```python
from build123d import *

# Parameters (mm, degrees)
F0_W      = 1200
F0_H      = 800
F1_DEPTH  = 60
F4_DEPTH  = 25
F5_W      = 1136.9413696229
F5_H      = 692.619483918
F6_DEPTH  = 30
F7_W      = 1159.0888965875
F7_H      = 738.1461262703
F8_DEPTH  = 15
F9_W      = 180.6832998991
F9_H      = 355.1081307232
F9_W_2    = 16.8206766248
F9_W_3    = 982.4556671083
F9_H_2    = 21.863527596
F9_H_3    = 568.6533860862
F10_DEPTH = 15


# Not quite as in the source:
# - the program builds the solid bodies; features that only make, move or delete a surface that nothing else refers to are left out


with BuildPart() as f1:
    # F0 (on Top) → F1 (new body)
    with BuildSketch(Plane.XY):
        with Locations((600, 400)):
            Rectangle(F0_W, F0_H)
    extrude(amount=F1_DEPTH)

    # F4 (add): a face of the model
    f4_faces = [f1.faces().sort_by_distance(p)[0] for p in [
        (600, 400, 0),
    ]]
    extrude(f4_faces, amount=F4_DEPTH)

    # F5 (on face) → F6 (cut)
    with BuildSketch(Plane(origin=(0, 0, -25), x_dir=(1, 0, 0), z_dir=(0, 0, -1))):
        with Locations((594.3454820663, -399.9507818371)):
            Rectangle(F5_W, F5_H)
    extrude(amount=-F6_DEPTH, mode=Mode.SUBTRACT)

    # F7 (on face) → F8 (cut)
    with BuildSketch(Plane.XY.offset(60)):
        with Locations((602.350092493, 395.9690630436)):
            Rectangle(F7_W, F7_H)
    extrude(amount=-F8_DEPTH, mode=Mode.SUBTRACT)

    # F9 (on face) → F10 (cut)
    with BuildSketch(Plane(origin=(0, 0, -25), x_dir=(1, 0, 0), z_dir=(0, 0, -1))):
        with Locations((-90.3416499496, -193.3716591448)):
            Rectangle(F9_W, F9_H)
        with Locations((8.4103383124, -193.3716591448)):
            Rectangle(F9_W_2, F9_H)
        with Locations((517.1026308089, -42.7092760801)):
            Rectangle(F9_W_3, F9_H_2)
        Polygon((1162.8161668777, -53.6410398781), (1008.3304643631, -53.6410398781), (1008.3304643631, -622.2944259644), (25.8747972548, -622.2944259644), (25.8747972548, -746.2605237961), (1162.8161668777, -746.2605237961), align=None)
        with Locations((517.1026308089, -337.9677329212)):
            Rectangle(F9_W_3, F9_H_3)
        Polygon((25.8747972548, -15.8175937831), (25.8747972548, -31.7775122821), (1008.3304643631, -31.7775122821), (1008.3304643631, -53.6410398781), (1162.8161668777, -53.6410398781), (1162.8161668777, -746.2605237961), (25.8747972548, -746.2605237961), (25.8747972548, -781.8935513496), (1179.8995733261, -781.8935513496), (1179.8995733261, -15.8175937831), align=None)
    extrude(amount=-F10_DEPTH, mode=Mode.SUBTRACT)


solid = f1.part
```
Check sheet for the modelled part. Datum: model origin and axes. Units: mm. A direction names the side the tool comes from. Give positions to 0.01 mm unless a question says otherwise; leave off trailing zeros. Order: outer loops, then holes, each group sorted by start corner. A loop starts at its lowest first (then second) coordinate and runs counter-clockwise, first axis right, second up. Notation, with made-up numbers: M -6,21 L 14,21 A25 ccw 14,47 Z; hole C 27.25,62 d1. An arc over 180 degrees is marked long. Answer in a Markdown table with one row per item. Add a question column.
Q1. Gauge pin test, flat ends, axial feed: pin 1 Ø7.5 at (y, z) = (231.5, -14) entering from -X; pin 2 Ø8 at (x, y) = (374.5, 261.5) entering from +Z. Record the tip position at first contact, or that the pin passes through.
Q2. Release check for a two-part mould opening along X. For faces 4 (the flat face through (592, 800, 18)), 5 (the flat face through (586, 395, 5)), 6 (the flat face through (25.875, 404, -10)), 7 (the flat face through (1200, 394, 18)) record: released by +X, released by -X, zero draft, split by the parting line, or undercut.
Q3. Thickness scan on L1, parallel to X at y = 310.5, z = -16; L2, parallel to X at y = 562, z = -14; L3, parallel to Y at x = 347, z = -19.5. Record the ranges inside material, lowest first.
Q4. Access from +Z, -Z, +X, -X, +Y, -Y to the whole of each face (thin tool, end or side, straight path). Record for faces 1 (the flat face through (331, 787, -25)), 2 (the flat face through (600, 28, -10)), 3 (the flat face through (594, 401, 45)).
Q5. Sectioned sample at B-B, the plane x = 456.5. Record the boundary of the cut face in (y, z).
Q6. Sectioned sample at A-A, the plane y = 496.5. Record the boundary of the cut face in (x, z), and give its area (3 significant figures).
Q7. Sectioned sample at C-C, the plane y = 87. Record the boundary of the cut face in (x, z), and give its area (3 significant figures).
Verdict:
| question | item | result |
|---|---|---|
| 1 | pin 1 | x = 16.82 |
| 1 | pin 2 | z = 45 |
| 2 | face 4 | zero draft |
| 2 | face 5 | undercut |
| 2 | face 6 | undercut |
| 2 | face 7 | released by +X |
| 3 | L1 | 16.82 to 25.87, 1179.9 to 1200 |
| 3 | L2 | 0 to 25.87, 1179.9 to 1200 |
| 3 | L3 | 0 to 15.82, 781.89 to 800 |
| 4 | face 1 | -Z, +X, -X, +Y, -Y |
| 4 | face 2 | -Z |
| 4 | face 3 | +Z |
| 5 | outline | M 0,-25 L 15.82,-25 L 15.82,-10 L 53.64,-10 L 53.64,5 L 746.26,5 L 746.26,-10 L 781.89,-10 L 781.89,-25 L 800,-25 L 800,60 L 765.04,60 L 765.04,45 L 26.9,45 L 26.9,60 L 0,60 Z |
| 6 | outline | M 0,-25 L 25.87,-25 L 25.87,5 L 1162.82,5 L 1162.82,-10 L 1179.9,-10 L 1179.9,-25 L 1200,-25 L 1200,60 L 1181.89,60 L 1181.89,45 L 22.81,45 L 22.81,60 L 0,60 Z |
| 6 | area | 50,200 mm² |
| 7 | outline | M 0,-10 L 16.82,-10 L 16.82,-25 L 25.87,-25 L 25.87,5 L 1162.82,5 L 1162.82,-10 L 1179.9,-10 L 1179.9,-25 L 1200,-25 L 1200,60 L 1181.89,60 L 1181.89,45 L 22.81,45 L 22.81,60 L 0,60 Z |
| 7 | area | 50,000 mm² |
